Could you check a few things on this model? Use its own coordinates, in mm. Round coordinates to 2 decimals unless told otherwise and drop trailing zeros. Loops run counter-clockwise (first coordinate to the right, second up) from the corner with the lowest first, then second, coordinate; pieces in that order, holes last. Notation, with made-up numbers: (-27, 25) -> (21, 25) arc R13 ccw to (21, 41) -> close; hole circle Ø4 at (-35, 64.25). An arc over 180 degrees is marked (long way). Put each result on its own line as item: value. Start each with the question number.
1. I need wall thicknesses on line 1 (X direction, y = -1.15, z = 96); line 2 (Z direction, x = 0, y = -2.05); line 3 (X direction, y = -1.85, z = -95.75). Which ranges of each line are inside material? Lowest first, please. Write a range as [from, to].
2. Imagine slicing it at A-A, the plane z = 71. Please give me the cut outline in (x, y), and give its area (3 significant figures).
3. I'm going to push a flat-ended pin straight in: P1, Ø3.5, axis at x = 0, z = -96, coming from the +Y side. Where does the tip first touch, or does it pass through?
4. Imagine slicing it at B-B, the plane x = -112. Please give me the cut outline in (y, z), and give its area (3 significant figures).
5. Imagine slicing it at C-C, the plane y = -2.3. Please give me the cut outline in (x, z).
```python
from build123d import *

# Parameters (mm, degrees)
F1_DEPTH = 3
F2_D     = 4.4


with BuildPart() as f1:
    # F0 (on Front) → F1 (new body)
    with BuildSketch(Plane.XZ):
        with BuildLine():
            Line((-131.25, -105.75), (131.25, -105.75))
            ThreePointArc((131.25, -105.75), (138.3210678119, -102.8210678119), (141.25, -95.75))
            Line((141.25, -95.75), (141.25, 95.75))
            ThreePointArc((141.25, 95.75), (138.3210678119, 102.8210678119), (131.25, 105.75))
            Line((131.25, 105.75), (-131.25, 105.75))
            ThreePointArc((-131.25, 105.75), (-138.3210678119, 102.8210678119), (-141.25, 95.75))
            Line((-141.25, 95.75), (-141.25, -95.75))
            ThreePointArc((-141.25, -95.75), (-138.3210678119, -102.8210678119), (-131.25, -105.75))
        make_face()
        with BuildLine():
            ThreePointArc((137.75, -74.25), (132.4779220614, -86.9779220614), (119.75, -92.25))
            Line((119.75, -92.25), (-119.75, -92.25))
            ThreePointArc((-119.75, -92.25), (-132.4779220614, -86.9779220614), (-137.75, -74.25))
            Line((-137.75, -74.25), (-137.75, 74.25))
            ThreePointArc((-137.75, 74.25), (-132.4779220614, 86.9779220614), (-119.75, 92.25))
            Line((-119.75, 92.25), (119.75, 92.25))
            ThreePointArc((119.75, 92.25), (132.4779220614, 86.9779220614), (137.75, 74.25))
            Line((137.75, 74.25), (137.75, -74.25))
        make_face(mode=Mode.SUBTRACT)
    extrude(amount=F1_DEPTH)

    # F2 (through all)
    with Locations(Plane(origin=(0, 0, 0), x_dir=(1, 0, 0), z_dir=(0, 1, 0))):
        with Locations((-131.5, -96), (0, -96), (131.5, -96), (131.25, 95.75), (0, 96), (-131.25, 95.75)):
            Hole(F2_D / 2)


solid = f1.part
```
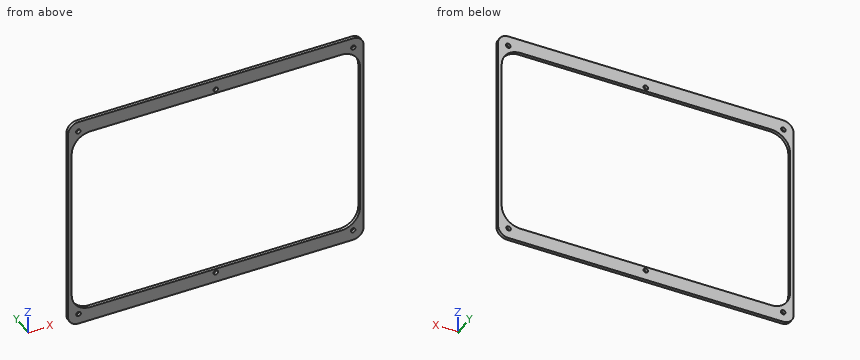
Entries:
1. line 1: [-141.25, -133.7], [-129.3, -2.2], [2.2, 129.3], [133.7, 141.25]
1. line 2: [-105.75, -98.2], [-93.8, -92.25], [92.25, 93.8], [98.2, 105.75]
1. line 3: [-141.25, -133.45], [-129.05, -2.19], [2.19, 129.05], [133.45, 141.25]
2. outline: (-141.25, -3) -> (-137.75, -3) -> (-137.75, 0) -> (-141.25, 0) -> close; (137.75, -3) -> (141.25, -3) -> (141.25, 0) -> (137.75, 0) -> close
2. area: 21.0 mm^2
3. P1: through
4. outline: (-3, -105.75) -> (0, -105.75) -> (0, -92.25) -> (-3, -92.25) -> close; (-3, 92.25) -> (0, 92.25) -> (0, 105.75) -> (-3, 105.75) -> close
4. area: 81.0 mm^2
5. outline: (-141.25, -95.75) arc R10 ccw to (-131.25, -105.75) -> (131.25, -105.75) arc R10 ccw to (141.25, -95.75) -> (141.25, 95.75) arc R10 ccw to (131.25, 105.75) -> (-131.25, 105.75) arc R10 ccw to (-141.25, 95.75) -> close; hole (-137.75, -74.25) arc R18 ccw to (-119.75, -92.25) -> (119.75, -92.25) arc R18 ccw to (137.75, -74.25) -> (137.75, 74.25) arc R18 ccw to (119.75, 92.25) -> (-119.75, 92.25) arc R18 ccw to (-137.75, 74.25) -> close; hole circle Ø4.4 at (-131.5, 96); hole circle Ø4.4 at (-131.25, -95.75); hole circle Ø4.4 at (0, -96); hole circle Ø4.4 at (0, 96); hole circle Ø4.4 at (131.25, -95.75); hole circle Ø4.4 at (131.5, 96)
